Build history of the part. All positions in model axes, mm. A direction names the side the tool comes from. Coordinates: 2 decimals unless noted, no trailing zeros. Write each loop counter-clockwise with the first axis right and the second up, starting at its lowest first coordinate (ties: lowest second). Pieces come first, ordered by that corner, then holes. Notation, with made-up numbers: (50.5, -25) -> (95.5, -25) arc R37 ccw to (95.5, 12) -> close; hole circle Ø5 at (45, 57.25). An arc over 180 degrees is marked (long way). Write each question's results on one line, items separated by ' | '. Start each with the question number.
Q1. Tool access for faces 4 (the face through (0, 4, 20)), 5 (the face through (-2, -15, 20)), 6 (the face through (8, 0, 3)): list every direction of +Z, -Z, +X, -X, +Y, -Y with a clear straight run to the whole face (end or side of a thin tool).
Q2. Saw through at D-D on z = 15.5. Give the cut face in (x, y).
Q3. Saw through at A-A on y = 9.5. Give the cut face in (x, z), and give its area (3 significant figures).
Q4. Two-plate mould, pull along Y, no slides. Class faces 1 (the face through (-13.36, 17.99, 19.72)), 2 (the face through (0, 0, 30)), 3 (the face through (-8, 0, 36)): released by +Y, released by -Y, zero draft, split by the parting line, or undercut.
Q5. Saw through at C-C on x = -10. Give the cut face in (y, z).
Q6. Saw through at B-B on x = -0.5. Give the cut face in (y, z).
Q7. Drill centre lines: line 1 (Z direction, x = 7.75, y = 2.5); line 2 (X direction, y = 4.5, z = 6); line 3 (Y direction, x = 1.25, z = 9). Where is each one in solid material? Low to high.
Q8. Drop flat-ended pins along their axis: pin 1 Ø3 at (x, z) = (-1, 9) entering from +Y; pin 2 Ø9 at (y, z) = (-14.5, 20.5) entering from -X; pin 3 Ø9 at (y, z) = (-14, 19.5) entering from +X. Give the stop position or say it passes through.
from build123d import *

# Parameters (mm, degrees)
PAD_DEPTH    = 40
SKETCH001_W  = 3
SKETCH001_H  = 5
POCKET_DEPTH = 28.701
CHAMFER_SIZE = 2


with BuildPart() as part:
    # Sketch → Pad (new body)
    with BuildSketch(Plane.XY):
        Polygon((-14.35, 19), (-11.35, 19), (-11.35, 4), (11.35, 4), (11.35, 19), (14.35, 19), (14.35, 0), (2, 0), (2, -30), (-2, -30), (-2, 0), (-14.35, 0), align=None)
    extrude(amount=PAD_DEPTH)

    # Sketch001 (on Face6 of Pad) → Pocket (cut, through all)
    with BuildSketch(Plane.YZ.offset(14.35)):
        with Locations((1.5, 30.5)):
            Rectangle(SKETCH001_W, SKETCH001_H)
        with Locations((1.5, 9.5)):
            Rectangle(SKETCH001_W, SKETCH001_H)
    extrude(amount=-POCKET_DEPTH, mode=Mode.SUBTRACT)

    # Chamfer
    chamfer_edges = [part.edges().sort_by_distance(p)[0] for p in [
        (-14.35, 19, 20),
        (14.35, 19, 20),
    ]]
    chamfer(chamfer_edges, length=CHAMFER_SIZE)


solid = part.part
Returned:
1) face 4: +Z, -Z, +Y | face 5: +Z, -Z, -X, -Y | face 6: +Z, -Z, +X, -Y
2) outline: (-14.35, 0) -> (-2, 0) -> (-2, -30) -> (2, -30) -> (2, 0) -> (14.35, 0) -> (14.35, 17) -> (12.35, 19) -> (11.35, 19) -> (11.35, 4) -> (-11.35, 4) -> (-11.35, 19) -> (-12.35, 19) -> (-14.35, 17) -> close
3) outline: (-14.35, 0) -> (-11.35, 0) -> (-11.35, 40) -> (-14.35, 40) -> close; (11.35, 0) -> (14.35, 0) -> (14.35, 40) -> (11.35, 40) -> close | area: 240 mm2
4) face 1: released by +Y | face 2: undercut | face 3: released by -Y
5) outline: (0, 0) -> (4, 0) -> (4, 40) -> (0, 40) -> (0, 33) -> (3, 33) -> (3, 28) -> (0, 28) -> (0, 12) -> (3, 12) -> (3, 7) -> (0, 7) -> close
6) outline: (-30, 0) -> (4, 0) -> (4, 40) -> (-30, 40) -> close; hole (0, 7) -> (3, 7) -> (3, 12) -> (0, 12) -> close; hole (0, 28) -> (3, 28) -> (3, 33) -> (0, 33) -> close
7) line 1: z = 0 to 7, 12 to 28, 33 to 40 | line 2: x = -14.35 to -11.35, 11.35 to 14.35 | line 3: y = -30 to 0, 3 to 4
8) pin 1: stops at y = 4 | pin 2: stops at x = -2 | pin 3: stops at x = 2
